Input: part model. Units: mm. Frame: model coordinates. A direction names the side the tool comes from. Give positions to 0.01 mm unless a question says otherwise; leave off trailing zeros. Loops run counter-clockwise (first coordinate to the right, second up) from the corner with the lowest first, then second, coordinate; pieces in that order, holes last. Notation, with made-up numbers: (-18, -29.75) -> (36, -29.75) arc R29 ccw to (36, 9.25) -> close; hole circle Ø3 at (33.5, 40.25). An arc over 180 degrees is marked (long way). One line per question, with ' | ' between items.
from build123d import *

# Parameters (mm, degrees)
SKETCH1_W                      = 96
SKETCH1_H                      = 96
BOSS_EXTRUDE1_DEPTH            = 8
SKETCH2_W                      = 92
SKETCH2_H                      = 92
COMPONENT_PLATFORM_DEPTH       = 6
CABLE_SLOTS_DEPTH              = 6
INNER_CORNER_FILLETS_R         = 3
M3X0_5_TAPPED_HOLE1_AT_2_COUNT = 2
M3X0_5_TAPPED_HOLE1_AT_2_PITCH = 70
M3X0_5_TAPPED_HOLE2_AT_2_COUNT = 2
M3X0_5_TAPPED_HOLE2_AT_2_PITCH = 70
M1_4X0_3_TAPPED_HOLE1_D        = 1.1
M1_4X0_3_TAPPED_HOLE1_DEPTH    = 3.7
M1_4X0_3_TAPPED_HOLE1_TIP      = 0.33047334
SKETCH29_R                     = 11
HDD_EXTRUSION_CUTOUT_DEPTH     = 10
HDD_EXTRUSION_CUTOUT_2_DEPTH   = 10
M3X0_5_TAPPED_HOLE3_D          = 2.5
M3X0_5_TAPPED_HOLE3_DEPTH      = 10
M3X0_5_TAPPED_HOLE3_TIP        = 0.751075774


with BuildPart() as part:
    # Sketch1 → Boss-Extrude1 (new body)
    with BuildSketch(Plane.XY):
        Rectangle(SKETCH1_W, SKETCH1_H)
    extrude(amount=BOSS_EXTRUDE1_DEPTH)

    # Sketch2 → Component Platform (cut)
    with BuildSketch(Plane.XY.offset(8)):
        Rectangle(SKETCH2_W, SKETCH2_H)
    extrude(amount=-COMPONENT_PLATFORM_DEPTH, mode=Mode.SUBTRACT)

    # Sketch3 → Cable Slots (cut, symmetric)
    with BuildSketch(Plane.XY.offset(2)):
        with BuildLine():
            Line((-33.878679656, -25.121320344), (-28.878679656, -20.121320344))
            ThreePointArc((-28.878679656, -20.121320344), (-28.228361402, -19.148050297), (-28, -18))
            Line((-28, -18), (-28, 18))
            ThreePointArc((-28, 18), (-28.228361402, 19.148050297), (-28.878679656, 20.121320344))
            Line((-28.878679656, 20.121320344), (-33.878679656, 25.121320344))
            ThreePointArc((-33.878679656, 25.121320344), (-34.851949703, 25.771638598), (-36, 26))
            Line((-36, 26), (-48, 26))
            Line((-48, 26), (-48, -26))
            Line((-48, -26), (-36, -26))
            ThreePointArc((-36, -26), (-34.851949703, -25.771638598), (-33.878679656, -25.121320344))
        make_face()
        with BuildLine():
            Line((48, -26), (48, 26))
            Line((48, 26), (36, 26))
            ThreePointArc((36, 26), (34.851949703, 25.771638598), (33.878679656, 25.121320344))
            Line((33.878679656, 25.121320344), (28.878679656, 20.121320344))
            ThreePointArc((28.878679656, 20.121320344), (28.228361402, 19.148050297), (28, 18))
            Line((28, 18), (28, -18))
            ThreePointArc((28, -18), (28.228361402, -19.148050297), (28.878679656, -20.121320344))
            Line((28.878679656, -20.121320344), (33.878679656, -25.121320344))
            ThreePointArc((33.878679656, -25.121320344), (34.851949703, -25.771638598), (36, -26))
            Line((36, -26), (48, -26))
        make_face()
    extrude(amount=CABLE_SLOTS_DEPTH, both=True, mode=Mode.SUBTRACT)

    # Inner Corner Fillets
    inner_corner_fillets_edges = [part.edges().sort_by_distance(p)[0] for p in [
        (-46, -46, 5),
        (-46, 46, 5),
        (46, 46, 5),
        (46, -46, 5),
    ]]
    fillet(inner_corner_fillets_edges, radius=INNER_CORNER_FILLETS_R)

    # Sketch14 → M3x0.5 Tapped Hole1 (revolve, cut)
    with BuildSketch(Plane(origin=(48, -35, 5), x_dir=(0, 0, -1), z_dir=(0, 1, 0))):
        Polygon((0, 0), (0, 10.751075774), (1.25, 10), (1.25, 0), align=None)
    m3x0_5_tapped_hole1 = revolve(axis=Axis((54.35, -35, 5), (-1, 0, 0)), mode=Mode.SUBTRACT)

    # M3x0.5 Tapped Hole1 at 2: M3x0.5 Tapped Hole1 ×2
    with Locations(*[(0, i * M3X0_5_TAPPED_HOLE1_AT_2_PITCH, 0) for i in range(1, M3X0_5_TAPPED_HOLE1_AT_2_COUNT)]):
        add(m3x0_5_tapped_hole1, mode=Mode.SUBTRACT)

    # Sketch16 → M3x0.5 Tapped Hole2 (revolve, cut)
    with BuildSketch(Plane(origin=(35, 48, 5), x_dir=(0, 0, 1), z_dir=(1, 0, 0))):
        Polygon((0, 0), (0, 10.751075774), (1.25, 10), (1.25, 0), align=None)
    m3x0_5_tapped_hole2 = revolve(axis=Axis((35, 54.35, 5), (0, -1, 0)), mode=Mode.SUBTRACT)

    # M3x0.5 Tapped Hole2 at 2: M3x0.5 Tapped Hole2 ×2
    with Locations(*[(-i * M3X0_5_TAPPED_HOLE2_AT_2_PITCH, 0, 0) for i in range(1, M3X0_5_TAPPED_HOLE2_AT_2_COUNT)]):
        add(m3x0_5_tapped_hole2, mode=Mode.SUBTRACT)

    # Mirror1: M3x0.5 Tapped Hole1 across plane
    add(m3x0_5_tapped_hole1.mirror(Plane(origin=(0, 0, 0), x_dir=(0, 0, 1), z_dir=(1, 0, 0))), mode=Mode.SUBTRACT)

    # Mirror1 copy 1 sketch → Mirror1 copy 1 (revolve, cut)
    with BuildSketch(Plane(origin=(-48, 35, 5), x_dir=(0, 0, -1), z_dir=(0, 1, 0))):
        Polygon((0, 0), (0, -10.751075774), (1.25, -10), (1.25, 0), align=None)
    revolve(axis=Axis((-54.35, 35, 5), (-1, 0, 0)), mode=Mode.SUBTRACT)

    # Mirror2: M3x0.5 Tapped Hole2 across plane
    add(m3x0_5_tapped_hole2.mirror(Plane(origin=(0, 0, 0), x_dir=(0, 0, 1), z_dir=(0, -1, 0))), mode=Mode.SUBTRACT)

    # Mirror2 copy 1 sketch → Mirror2 copy 1 (revolve, cut)
    with BuildSketch(Plane(origin=(-35, -48, 5), x_dir=(0, 0, 1), z_dir=(1, 0, 0))):
        Polygon((0, 0), (0, -10.751075774), (1.25, -10), (1.25, 0), align=None)
    revolve(axis=Axis((-35, -54.35, 5), (0, -1, 0)), mode=Mode.SUBTRACT)

    # M1.4x0.3 Tapped Hole1
    with Locations(Plane.XY.offset(2)):
        with Locations((-19.31998517, -29.75), (24.78001483, -32.85), (24.78001483, 32.85), (-22.91998517, 32.85)):
            Hole(M1_4X0_3_TAPPED_HOLE1_D / 2, depth=M1_4X0_3_TAPPED_HOLE1_DEPTH)
            with Locations((0, 0, -(M1_4X0_3_TAPPED_HOLE1_DEPTH + M1_4X0_3_TAPPED_HOLE1_TIP / 2))):  # 118° drill point
                Cone(0, M1_4X0_3_TAPPED_HOLE1_D / 2, M1_4X0_3_TAPPED_HOLE1_TIP, mode=Mode.SUBTRACT)

    # Sketch29 → HDD Extrusion Cutout (cut)
    with BuildSketch(Plane(origin=(0, 0, 0), x_dir=(-1, 0, 0), z_dir=(0, 0, -1))):
        with Locations((-0.08192631, -8.74785827)):
            Circle(SKETCH29_R)
    extrude(amount=-HDD_EXTRUSION_CUTOUT_DEPTH, mode=Mode.SUBTRACT)

    # Sketch9 → HDD Extrusion Cutout 2 (cut)
    with BuildSketch(Plane.XY.offset(2)):
        with BuildLine():
            Line((24.08001483, 32.25), (24.08001483, 15.25))
            Line((24.08001483, 15.25), (19.08001483, 15.25))
            ThreePointArc((19.08001483, 15.25), (10.594733456, 18.764718626), (7.08001483, 27.25))
            Line((7.08001483, 27.25), (7.08001483, 32.25))
            Line((7.08001483, 32.25), (24.08001483, 32.25))
        make_face()
    extrude(amount=-HDD_EXTRUSION_CUTOUT_2_DEPTH, mode=Mode.SUBTRACT)

    # M3x0.5 Tapped Hole3
    with Locations(Plane.XY.offset(2)):
        with Locations((-30.20998517, -37.56), (29.79001483, -37.56), (29.79001483, 37.44), (-30.20998517, 37.44)):
            Hole(M3X0_5_TAPPED_HOLE3_D / 2, depth=M3X0_5_TAPPED_HOLE3_DEPTH)
            with Locations((0, 0, -(M3X0_5_TAPPED_HOLE3_DEPTH + M3X0_5_TAPPED_HOLE3_TIP / 2))):  # 118° drill point
                Cone(0, M3X0_5_TAPPED_HOLE3_D / 2, M3X0_5_TAPPED_HOLE3_TIP, mode=Mode.SUBTRACT)


solid = part.part
1. Section query C-C (y = -7.5). Output: boundary loops of the cut face in (x, z), then the cut area to 3 significant figures.
Determined:
outline: (-28, 0) -> (-10.85, 0) -> (-10.85, 2) -> (-28, 2) -> close; (11.01, 0) -> (28, 0) -> (28, 2) -> (11.01, 2) -> close | area: 68.3 mm2
2. Reachability of faces 1 (the flat face through (-45, -26, 1)), 2 (the cylindrical face through (-47.01, -33.78, 5.27)), 3 (the cylindrical face through (10.69, 18.67, 1.01)), 4 (the flat face through (46, -34.6, 6.4)) from +Z, -Z, +X, -X, +Y, -Y: full face, straight path, thin tool, end or side. Return the list, or none.
Determined:
face 1: +Z, -Z, -X | face 2: +X, -X | face 3: +Z, -Z | face 4: +Z
3. Pin query (flat end, axial travel): P1, Ø2, axis at y = 35, z = 5, coming from the +X side; P2, Ø1.4, axis at x = -19.32, y = -29.75, coming from the +Z side; P3, Ø3, axis at x = 35, z = 5, coming from the -Y side; P4, Ø2, axis at y = -3.5, z = 1, coming from the -X side. Return the tip coordinate at first contact, or that it passes through.
Determined:
P1: passes through | P2: stops at z = 2 | P3: stops at y = -48 | P4: stops at x = -28
4. Section query A-A (y = 35). Output: boundary loops of the cut face in (x, z).
Determined:
outline: (-48, 0) -> (48, 0) -> (48, 3.75) -> (46, 3.75) -> (46, 2) -> (-46, 2) -> (-46, 3.75) -> (-48, 3.75) -> close; (-48, 6.25) -> (-46, 6.25) -> (-46, 8) -> (-48, 8) -> close; (46, 6.25) -> (48, 6.25) -> (48, 8) -> (46, 8) -> close
5. Pull-direction query (X, two-part tool) for faces 5 (the flat face through (48, -37, 4)), 6 (the cylindrical face through (-30.05, 38.68, 0.99)), 7 (the flat face through (-48, 37, 4)); classes: pulls with the +X half, pulls with the -X half, needs draft (parallel to the pull), parting line crosses it, or undercut.
Determined:
face 5: pulls with the +X half | face 6: undercut | face 7: pulls with the -X half
6. Section query B-B (x = -37.5). Output: boundary loops of the cut face in (y, z).
Determined:
outline: (-48, 0) -> (-26, 0) -> (-26, 2) -> (-46, 2) -> (-46, 8) -> (-48, 8) -> close; (26, 0) -> (48, 0) -> (48, 8) -> (46, 8) -> (46, 2) -> (26, 2) -> close
7. Section query D-D (z = 5). Count the separate pieces of the cut face and the enclosed holes in it, then the cut area to 3 significant figures.
Determined:
separate pieces: 10 | enclosed holes: 0 | area: 512 mm2
8. Ray query, line 1 along X through (y, z) = (-46.95, 5); line 2 along Y through (x, z) = (-46.55, 5); line 3 along X through (y, z) = (32.85, 0.55). Return the intervals inside material, ascending. Write a range as from..to.
Determined:
line 1: x = -48..-36.25, -33.75..33.75, 36.25..48 | line 2: y = -48..-36.25, -33.75..-26, 26..33.75, 36.25..48 | line 3: x = -48..-23.47, -22.37..24.23, 25.33..48
